Could you check a few things on this model? Use its own coordinates, in mm. A direction names the side the tool comes from. Give positions to 0.01 mm unless a question says otherwise; leave off trailing zeros. Loops run counter-clockwise (first coordinate to the right, second up) from the corner with the lowest first, then second, coordinate; pieces in that order, holes last.
1. For faces 4 (the flat face through (0, 15.2, 10.5)), 5 (the cylindrical face through (-4.041, 14.79, -7.986)), 6 (the cylindrical face through (10.514, 12.957, 0.651)), 7 (the flat face through (0, 15.2, -10.4)), which set-ups out of +Z, -Z, +X, -X, +Y, -Y let a thin tool reach every point of the face, with its end or its side?
2. I need wall thicknesses on line 1 along Y through (x, z) = (10.25, 0); line 2 along Z through (x, y) = (9.9, 22); line 3 along X through (y, z) = (27.25, 6.5). Which ranges of each line are inside material? Lowest first, please.
3. Imagine slicing it at B-B (z = 0). List the corners of the cut face in (x, y) for me, plus the area to 3 significant figures.
4. Imagine slicing it at A-A (x = -7.5). List the corners of the cut face in (y, z) for me, plus the area to 3 significant figures.
5. Thinking about a two-plate mould opening in X: for faces 1 (the cylindrical face through (10.51, 17.12, 1.08)), 2 (the cylindrical face through (8.948, 15.21, 0.197)), 3 (the flat face through (9.5, 22, 0)), which applies, +X half, -X half, draft (parallel to the pull), parting line (faces both ways), or undercut?
6. Imagine slicing it at D-D (x = 1.25). List the corners of the cut face in (y, z) for me, plus the area to 3 significant figures.
7. For P1, Ø3, axis at y = 10, z = -1, coming from the +X side; P2, Ø9, axis at y = 8, z = 0, coming from the -X side; P3, Ø1, axis at x = 4.5, z = -7, coming from the -Y side, each with a flat end and sliding along its axis, tell me the tip position at first contact or that it passes through.
Autodesk Inventor part; units mm, degrees
ref_plane "YZ Plane" through (0, 0, 0) normal (1, 0, 0) x (0, 1, 0)
ref_plane "XZ Plane" through (0, 0, 0) normal (0, 1, 0) x (-1, 0, 0)
ref_plane "XY Plane" through (0, 0, 0) normal (0, 0, 1) x (1, 0, 0)
sketch "Эскиз1" plane through (0, 0, 0) normal (0, 1, 0) x (-1, 0, 0)
  circle A0 centre (0, 0) radius 8.95
  circle A1 centre (0, 0) radius 9.95
  line L0 (0, 0) -> (7.9399, 5.9967)
  line L1 (0, 0) -> (7.9399, -5.9967)
  point P0 (7.1419, -5.394)
  point P1 (7.1419, 5.394)
  dimension "d0" = 17.9
  dimension "d1" = 19.9
extrude "Выдавливание1" add sketch "Эскиз1" along normal blind 30 contours A0 L1 A1 L0 picked at (-8.7459, -3.8334)
sketch "Эскиз2" plane through (0, 30, 0) normal (0, 1, 0) x (1, 0, 0)
  arc A0 (-7.1419, -5.394) -> (-8.0346, -4.8641) centre (-9.8432, -8.9279) ccw
  arc A1 (-8.0346, -4.8641) -> (-9.1915, -6.6699) centre (-8.4689, -5.8593) ccw
  line L0 (-9.1915, -6.6699) -> (-8.5202, -5.8154)
  arc A2 (-7.9413, -5.9822) -> (-8.5202, -5.8154) centre (-8.3096, -6.1726) ccw
  line L1 (-7.1419, -5.394) -> (-7.9399, -5.9967)
  line L2 (-7.9399, -5.9967) -> (-7.1419, -5.394)
  line L3 (-7.9399, -5.9967) -> (-7.9413, -5.9822)
  line L4 (-0.0151, 0) -> (-3.489, 0)
  arc A3 (-8.0346, 4.8641) -> (-7.1419, 5.394) centre (-9.8432, 8.9279) ccw
  arc A4 (-8.5202, 5.8154) -> (-7.9413, 5.9822) centre (-8.3096, 6.1726) ccw
  line L5 (-7.1419, 5.394) -> (-7.9399, 5.9967)
  line L6 (-7.9399, 5.9967) -> (-7.1419, 5.394)
  line L7 (-7.9399, 5.9967) -> (-7.9413, 5.9822)
  arc A5 (-9.1915, 6.6699) -> (-8.0346, 4.8641) centre (-8.4689, 5.8593) ccw
  line L8 (-9.1915, 6.6699) -> (-8.5202, 5.8154)
  point P0 (-7.1419, 5.394)
  point P1 (-7.9399, -5.9967)
  point P2 (-5.3694, -4.0591)
  point P3 (-7.9399, 5.9967)
  point P4 (-5.3694, 4.0591)
  point P5 (-7.9399, 5.9967)
  dimension "d25" = 1.0859
sketch "Эскиз3" plane through (0, 30, 0) normal (0, 1, 0) x (1, 0, 0)
  arc A0 (-7.9399, -5.9967) -> (-7.9399, 5.9967) centre (0, 0) ccw
  line L0 (11.5, -6.95) -> (11.5, 6.95)
  arc A1 (-7.1419, -5.394) -> (-7.1419, 5.394) centre (0, 0) ccw
  arc A2 (0, -8.95) -> (0, 8.95) centre (0, 0) ccw
  line L1 (0, -9.95) -> (0, -8.95)
  line L2 (0, 8.95) -> (0, 9.95)
  line L3 (11.5, 6.95) -> (11.5, 10.95)
  line L4 (11.5, -6.95) -> (11.5, -10.95)
  line L5 (0, 5.45) -> (0, 9.95)
  line L6 (11.5, -10.95) -> (0, -10.95)
  line L7 (0, -10.95) -> (0, -9.95)
  line L8 (11.5, 10.95) -> (0, 10.95)
  line L9 (0, 10.95) -> (0, 9.95)
  point P0 (0, 8.95)
  dimension "d13" = 4
  dimension "d14" = 4
  dimension "d22" = 21.9
  dimension "d23" = 2
extrude "Выдавливание3" add sketch "Эскиз3" against normal blind 30
ref_plane "РабПлоскость1" through (11.5, 20, 4.95) normal (1, 0, 0) x (0, 0, -1)
sketch "Эскиз4" plane through (11.5, 20, 4.95) normal (1, 0, 0) x (0, 0, -1)
  line L0 (4.95, -20) -> (4.95, 10)
  line L1 (1, 10) -> (8.9, 10)
  circle A0 centre (4.95, -12) radius 5
  line L2 (14.4, -20) -> (-4.5, -20)
  circle A1 centre (4.95, 2) radius 5
  line L3 (-4.5, 10) -> (14.4, 10)
  point P0 (7.3306, 10)
  point P1 (2.5694, 10)
  point P2 (4.95, 10)
  dimension "d15" = 10
  dimension "d16" = 8
  dimension "d17" = 10
  dimension "d18" = 8
extrude "Выдавливание4" cut sketch "Эскиз4" against normal blind 2
extrude "Выдавливание5" add sketch "Эскиз2" against normal blind 30
properties part number "крепление маркера 18мм"
Derived:
1. face 4: +Z, -X, +Y, -Y
1. face 5: +Y, -Y
1. face 6: +X
1. face 7: -Z, -X, +Y, -Y
2. line 1: y = 0 to 3, 13 to 17, 27 to 30
2. line 2: z = -10.95 to -5, 5 to 10.95
2. line 3: x = -9.35 to -9.06, -7.53 to -6.15, 6.15 to 11.5
3. outline: (8.95, 0) - (11.5, 0) - (11.5, 3) - (9.5, 3) - (9.5, 13) - (11.5, 13) - (11.5, 17) - (9.5, 17) - (9.5, 27) - (11.5, 27) - (11.5, 30) - (8.95, 30) - close
3. area: 36.5 mm2
4. outline: (0, -6.54) - (30, -6.54) - (30, -5.15) - (0, -5.15) - close; (0, 5.15) - (30, 5.15) - (30, 6.54) - (0, 6.54) - close
4. area: 83.5 mm2
5. face 1: draft
5. face 2: undercut
5. face 3: +X half
6. outline: (0, -10.95) - (30, -10.95) - (30, -8.86) - (0, -8.86) - close; (0, 8.86) - (30, 8.86) - (30, 10.95) - (0, 10.95) - close
6. area: 125 mm2
7. P1: stops at x = 9.5
7. P2: stops at x = 7.74
7. P3: passes through
